Part model, mm, in its own coordinate system. A direction names the side the tool comes from. Coordinates: 2 decimals unless noted, no trailing zeros. Loops run counter-clockwise (first coordinate to the right, second up) from the corner with the lowest first, then second, coordinate; pieces in that order, holes last. Notation, with made-up numbers: (-29.75, 38.25) - (-24.75, 38.25) arc R11 cw to (-24.75, 43.25) - close; hole circle Ø3 at (-38, 81). An arc over 180 degrees is marked (long way). Use a Markdown table: item, result. Add a question column.
1) Pull direction Z, two halves, no side cores. Call faces 1 (the face through (0, 0, 6)), 2 (the face through (14.37, 7.81, -1.73)), 3 (the face through (12.68, -3.04, -3.32)): +Z half, -Z half, draft (parallel to the pull), parting line (faces both ways), or undercut.
2) Band-saw the part on C-C (x = 23). Give the cut face in (y, z), plus the area to 3 significant figures.
3) Tool access for faces 4 (the face through (5, -6, -6)), 5 (the face through (2, -12, -2)), 6 (the face through (2.46, 12.99, -0.54)): list every direction of +Z, -Z, +X, -X, +Y, -Y with a clear straight run to the whole face (end or side of a thin tool).
4) Drop flat-ended pins along their axis: P1, Ø4, axis at x = 11.5, y = -3.5, coming from the -Z side; P2, Ø1, axis at x = 11.5, y = 0, coming from the -Z side; P3, Ø1, axis at x = 12.5, z = -2, coming from the -Y side; P4, Ø5, axis at x = 4.5, z = -1, coming from the -Y side. Give the stop position or say it passes through.
5) Band-saw the part on A-A (y = 0). Give the cut face in (x, z), plus the area to 3 significant figures.
6) Probe probe 1 along Y at (x, z) = (13.25, 0); probe 2 along X at (y, z) = (-4.5, -7.75); probe 3 along Y at (x, z) = (19, -2.5). List the from-to ranges inside material, lowest first. Write a range as [from, to].
7) Band-saw the part on B-B (z = 0). Give the cut face in (x, y), plus the area to 3 significant figures.
8) Band-saw the part on D-D (y = -10.25). Give the cut face in (x, z).
from build123d import *

# Parameters (mm, degrees)
CHANFREIN2_SIZE         = 1
ENL_V_MAT_EXTRU_1_DEPTH = 32.032241298


with BuildPart() as part:
    # Esquisse1 → Base-Révolution (revolve)
    with BuildSketch(Plane.XY, mode=Mode.PRIVATE) as base_r_volution_sk:
        Polygon((0, 4.5), (25, 4.5), (25, 8), (5, 8), (5, 13), (0, 13), align=None)
    revolve(base_r_volution_sk.sketch.rotate(Axis((0, 0, 0), (1, 0, 0)), 90), axis=Axis((0, 0, 0), (1, 0, 0)))

    # Chanfrein2
    chanfrein2_edges = [part.edges().sort_by_distance(p)[0] for p in [
        (25, 0, -8),
    ]]
    chamfer(chanfrein2_edges, length=CHANFREIN2_SIZE)

    # Esquisse2 → Enlèv. mat.-Extru.1 (cut, through all)
    with BuildSketch(Plane.ZY):
        with BuildLine():
            Line((2, -11), (2, -12.845232579))
            ThreePointArc((2, -12.845232579), (0, -13), (-2, -12.845232579))
            Line((-2, -12.845232579), (-2, -11))
            ThreePointArc((-2, -11), (0, -9), (2, -11))
        make_face()
    extrude(amount=-ENL_V_MAT_EXTRU_1_DEPTH, mode=Mode.SUBTRACT)


solid = part.part
Answer block:
| question | item | result |
|---|---|---|
| 1 | face 1 | draft |
| 1 | face 2 | parting line |
| 1 | face 3 | undercut |
| 2 | outline | circle Ø16 at (0, 0); hole circle Ø9 at (0, 0) |
| 2 | area | 137 mm2 |
| 3 | face 4 | +X |
| 3 | face 5 | +X, -X, -Y |
| 3 | face 6 | +X, -X |
| 4 | P1 | z = -7.86 |
| 4 | P2 | z = -8 |
| 4 | P3 | y = -7.86 |
| 4 | P4 | y = -12.85 |
| 5 | outline | (0, -13) - (5, -13) - (5, -8) - (24, -8) - (25, -7) - (25, -4.5) - (0, -4.5) - close; (0, 4.5) - (25, 4.5) - (25, 7) - (24, 8) - (5, 8) - (5, 13) - (0, 13) - close |
| 5 | area | 224 mm2 |
| 6 | probe 1 | [-8, -4.5], [4.5, 8] |
| 6 | probe 2 | [0, 5] |
| 6 | probe 3 | [-7.6, -3.74], [3.74, 7.6] |
| 7 | outline | (0, -9) - (5, -9) - (5, -8) - (24, -8) - (25, -7) - (25, -4.5) - (0, -4.5) - close; (0, 4.5) - (25, 4.5) - (25, 7) - (24, 8) - (5, 8) - (5, 13) - (0, 13) - close |
| 7 | area | 204 mm2 |
| 8 | outline | (0, -8) - (5, -8) - (5, -1.85) - (0, -1.85) - close; (0, 1.85) - (5, 1.85) - (5, 8) - (0, 8) - close |
